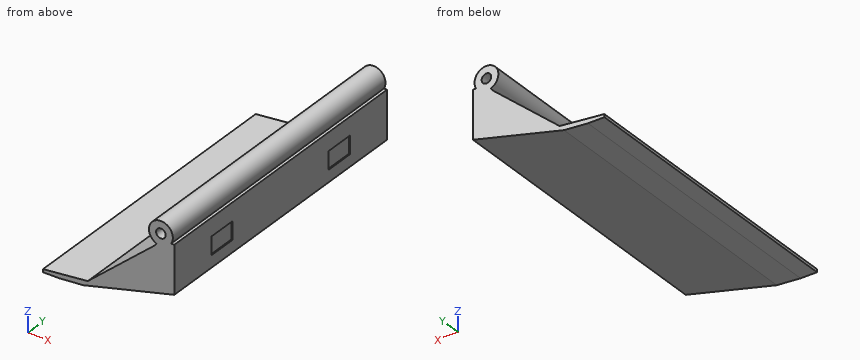
from build123d import *

# Parameters (mm, degrees)
ONE_PIECE_PROGRESSIVE_SOLID_WEDGE_DEPTH      = 99.7
ONE_PIECE_PROGRESSIVE_SOLID_WEDGE_DEPTH_BACK = 99.7
INTEGRAL_FULL_WIDTH_PIVOT_BOSS_DEPTH         = 99.7
INTEGRAL_FULL_WIDTH_PIVOT_BOSS_DEPTH_BACK    = 99.7
SKETCH_2_R                                   = 8
M6_MANUAL_PIVOT_DEPTH                        = 110
M6_MANUAL_PIVOT_DEPTH_BACK                   = 110
SKETCH_3_R                                   = 3.2
RECESSED_HOOK_PATCH_65_START                 = -45
SKETCH_4_W                                   = 0.81
SKETCH_4_H                                   = 12
RECESSED_HOOK_PATCH_65_DEPTH                 = 20
RECESSED_HOOK_PATCH_45_START                 = 65
SKETCH_5_W                                   = 0.81
SKETCH_5_H                                   = 12
RECESSED_HOOK_PATCH_45_DEPTH                 = 20


with BuildPart() as part:
    # Sketch 1 → One_piece_progressive_solid_wedge (new, two sides: drawn at the far end of the back side and taken through both)
    with BuildSketch(Plane(origin=(0, 0, 0), x_dir=(1, 0, 0), z_dir=(0, 1, 0)).offset(-ONE_PIECE_PROGRESSIVE_SOLID_WEDGE_DEPTH_BACK)):
        Polygon((-198, -1.2), (-198, -3.2), (-168, -6.2), (-123, -45), (-119, -50), (-110, -50), (-110, -18), (-171, -2.5), (-187, -1.2), align=None)
    extrude(amount=ONE_PIECE_PROGRESSIVE_SOLID_WEDGE_DEPTH + ONE_PIECE_PROGRESSIVE_SOLID_WEDGE_DEPTH_BACK)

    # Sketch 2 → Integral_full_width_pivot_boss (add, two sides: drawn at the far end of the back side and taken through both)
    with BuildSketch(Plane(origin=(0, 0, 0), x_dir=(1, 0, 0), z_dir=(0, 1, 0)).offset(-INTEGRAL_FULL_WIDTH_PIVOT_BOSS_DEPTH_BACK)):
        with Locations((-119, -54)):
            Circle(SKETCH_2_R)
    extrude(amount=INTEGRAL_FULL_WIDTH_PIVOT_BOSS_DEPTH + INTEGRAL_FULL_WIDTH_PIVOT_BOSS_DEPTH_BACK)

    # Sketch 3 → M6_manual_pivot (cut, two sides: drawn at the far end of the back side and taken through both)
    with BuildSketch(Plane(origin=(0, 0, 0), x_dir=(1, 0, 0), z_dir=(0, 1, 0)).offset(-M6_MANUAL_PIVOT_DEPTH_BACK)):
        with Locations(Location((-119, -54, 0), (0, 0, 270))):
            Circle(SKETCH_3_R)
    extrude(amount=M6_MANUAL_PIVOT_DEPTH + M6_MANUAL_PIVOT_DEPTH_BACK, mode=Mode.SUBTRACT)

    # Sketch 4 → Recessed_hook_patch_-65 (cut)
    with BuildSketch(Plane(origin=(0, 0, 0), x_dir=(1, 0, 0), z_dir=(0, 1, 0)).offset(RECESSED_HOOK_PATCH_65_START)):
        with Locations((-110.395, -32)):
            Rectangle(SKETCH_4_W, SKETCH_4_H)
    extrude(amount=-RECESSED_HOOK_PATCH_65_DEPTH, mode=Mode.SUBTRACT)

    # Sketch 5 → Recessed_hook_patch_45 (cut)
    with BuildSketch(Plane(origin=(0, 0, 0), x_dir=(1, 0, 0), z_dir=(0, 1, 0)).offset(RECESSED_HOOK_PATCH_45_START)):
        with Locations((-110.395, -32)):
            Rectangle(SKETCH_5_W, SKETCH_5_H)
    extrude(amount=-RECESSED_HOOK_PATCH_45_DEPTH, mode=Mode.SUBTRACT)


solid = part.part
The listing builds one solid part. Answer for the finished solid, in the listing's coordinates (mm). Give positions to 0.01 mm unless a question says otherwise; leave off trailing zeros. Loops run counter-clockwise (first coordinate to the right, second up) from the corner with the lowest first, then second, coordinate; pieces in that order, holes last. Notation, with made-up numbers: (83.5, 5) - (122.5, 5) arc R29 ccw to (122.5, 38) - close; hole circle Ø7 at (9.5, 77.5). An arc over 180 degrees is marked (long way). Answer as a JSON object with one key per item and string values.
1. A cutting plane is placed at A-A (z = 54). Write down the section's boundary in (x, y), then the cut area to 3 significant figures.
Determined:
{"outline": "(-127, -99.7) - (-122.2, -99.7) - (-122.2, 99.7) - (-127, 99.7) - close; (-115.8, -99.7) - (-111, -99.7) - (-111, 99.7) - (-115.8, 99.7) - close", "area": "1,910 mm²"}
2. Flat-ended cylindrical pins translate along their axes: pin 1 Ø13 at (y, z) = (-59.5, 35) entering from +X; pin 2 Ø1 at (y, z) = (53, 52.5) entering from +X; pin 3 Ø0.6 at (x, y) = (-110.5, -58.5) entering from -Z; pin 4 Ø2 at (x, y) = (-127, -30.5) entering from -Z. Find the tip coordinate at first contact, or state that the pin passes through.
Determined:
{"pin 1": "x = -110", "pin 2": "x = -111.06", "pin 3": "z = 17.8", "pin 4": "z = 13.43"}
3. A cutting plane is placed at B-B (y = -78). Write down the section's boundary in (x, z), then the cut area to 3 significant figures.
Determined:
{"outline": "(-198, 1.2) - (-187, 1.2) - (-171, 2.5) - (-110, 18) - (-110, 50) - (-112.07, 50) arc R8 ccw (long way) to (-121.8, 46.5) - (-123, 45) - (-168, 6.2) - (-198, 3.2) - close; hole circle Ø6.4 at (-119, 54)", "area": "1,410 mm²"}
4. A cutting plane is placed at C-C (x = -119). Write down the section's boundary in (y, z).
Determined:
{"outline": "(-99.7, 15.71) - (99.7, 15.71) - (99.7, 50.8) - (-99.7, 50.8) - close; (-99.7, 57.2) - (99.7, 57.2) - (99.7, 62) - (-99.7, 62) - close"}
5. Find the intervals of material crossed by L1, parallel to X at y = 19, z = 54; L2, parallel to Z at x = -119, y = 0; L3, parallel to Z at x = -116.5, y = 35, in increasing order. Write a range as [from, to].
Determined:
{"L1": "[-127, -122.2], [-115.8, -111]", "L2": "[15.71, 50.8], [57.2, 62]", "L3": "[16.35, 52], [56, 61.6]"}
6. A cutting plane is placed at D-D (z = 33.5). Write down the section's boundary in (x, y), then the cut area to 3 significant figures.
Determined:
{"outline": "(-136.34, -99.7) - (-110, -99.7) - (-110, -65) - (-110.8, -65) - (-110.8, -45) - (-110, -45) - (-110, 45) - (-110.8, 45) - (-110.8, 65) - (-110, 65) - (-110, 99.7) - (-136.34, 99.7) - close", "area": "5,220 mm²"}
